Answer from the drawing. Dimensions are ordinates in mm from the lowest x, y and z of the part. A direction names the side the tool comes from. Coordinates: 2 decimals unless noted, no trailing zeros. Write each loop counter-clockwise with the first axis right and the second up, starting at its lowest first coordinate (ties: lowest second). Pieces come first, ordered by that corner, then holes. Notation, with made-up numbers: (13, 57.5) -> (52, 57.5) arc R6 ccw to (52, 66.5) -> close; hole circle Ø3 at (-4.5, 57.5). An arc over 180 degrees is marked (long way). One line per item, written item: value. Start each with the question number.
1. For a pull along X with two mould halves and no side action, classify the marked faces 6, 7 and 8 as pulls with the +X half, pulls with the -X half, needs draft (parallel to the pull), parting line crosses it, or undercut.
2. For the marked faces 1, 2, 3, 4 and 5, determine the directions among +Z, -Z, +X, -X, +Y, -Y from which every point of the face is accessible in a straight line to the end or side of a thin tool.
3. Find section B-B, the plane x = 110. Write down the section's boundary in (y, z), and give its area (3 significant figures).
4. Find section A-A, the plane z = 27. Write down the section's boundary in (x, y), and give its area (3 significant figures).
5. Consider line 1 along Y through (x, z) = (110, 59); line 2 along Y through (x, z) = (110, 9); line 3 along Y through (x, z) = (85, 51). Determine where each line is inside the solid, lowest interval first.
6. Given P1, Ø16, axis at x = 110, y = 45, coming from the +Z side; P2, Ø5, axis at x = 32.5, y = 61, coming from the +Z side; P3, Ø12, axis at x = 96, y = 72, coming from the +Z side, each flat-ended and moving along its own axis, determine where each tip first touches the part or whether it passes through.
7. Find section C-C, the plane y = 30. Write down the section's boundary in (x, z).
8. Find section D-D, the plane z = 62.5. Write down the section's boundary in (x, y).
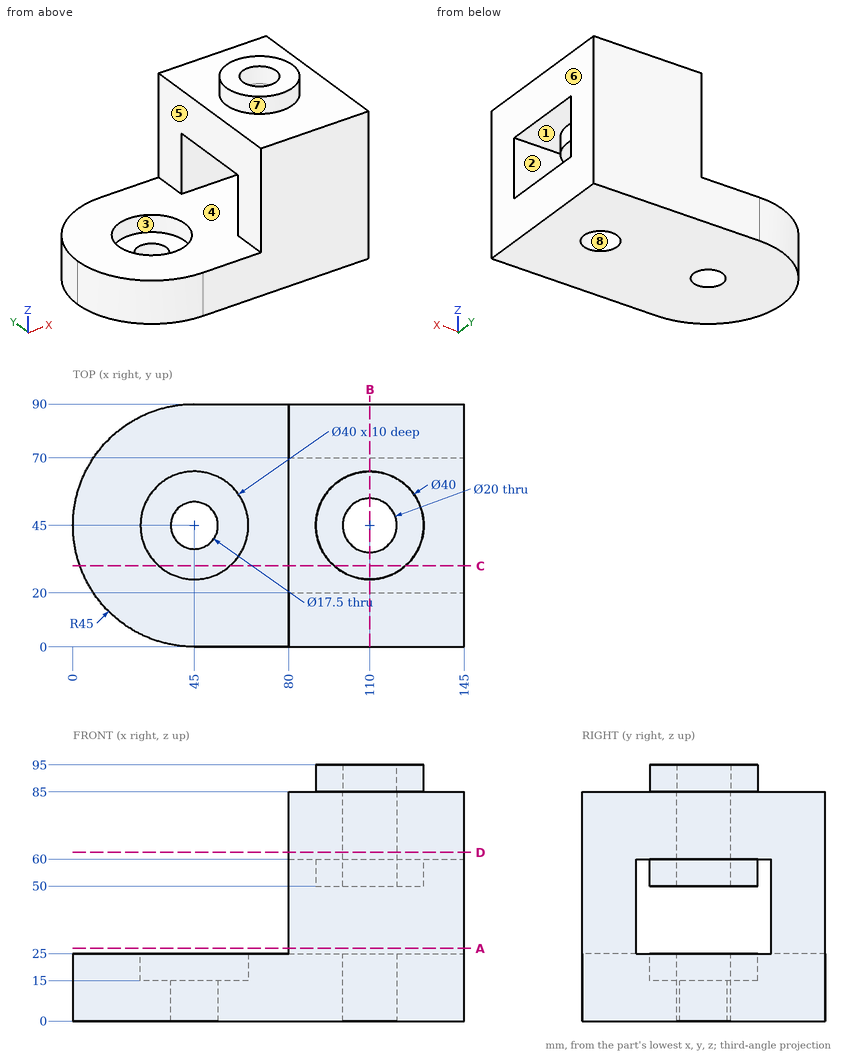
Answer block:
1. face 6: pulls with the +X half
1. face 7: parting line crosses it
1. face 8: undercut
2. face 1: none
2. face 2: +X, -X
2. face 3: +Z
2. face 4: -X
2. face 5: +Z, -X, +Y, -Y
3. outline: (0, 0) -> (35, 0) -> (35, 25) -> (20, 25) -> (20, 60) -> (25, 60) -> (25, 50) -> (35, 50) -> (35, 95) -> (25, 95) -> (25, 85) -> (0, 85) -> close; (55, 0) -> (90, 0) -> (90, 85) -> (65, 85) -> (65, 95) -> (55, 95) -> (55, 50) -> (65, 50) -> (65, 60) -> (70, 60) -> (70, 25) -> (55, 25) -> close
3. area: 5,300 mm2
4. outline: (80, 0) -> (145, 0) -> (145, 20) -> (80, 20) -> close; (80, 70) -> (145, 70) -> (145, 90) -> (80, 90) -> close
4. area: 2,600 mm2
5. line 1: y = 0 to 20, 25 to 35, 55 to 65, 70 to 90
5. line 2: y = 0 to 35, 55 to 90
5. line 3: y = 0 to 20, 70 to 90
6. P1: passes through
6. P2: stops at z = 25
6. P3: stops at z = 85
7. outline: (2.57, 0) -> (145, 0) -> (145, 25) -> (58.23, 25) -> (58.23, 15) -> (31.77, 15) -> (31.77, 25) -> (2.57, 25) -> close; (80, 60) -> (96.77, 60) -> (96.77, 50) -> (123.23, 50) -> (123.23, 60) -> (145, 60) -> (145, 85) -> (123.23, 85) -> (123.23, 95) -> (96.77, 95) -> (96.77, 85) -> (80, 85) -> close
8. outline: (80, 0) -> (145, 0) -> (145, 90) -> (80, 90) -> close; hole circle Ø20 at (110, 45)
